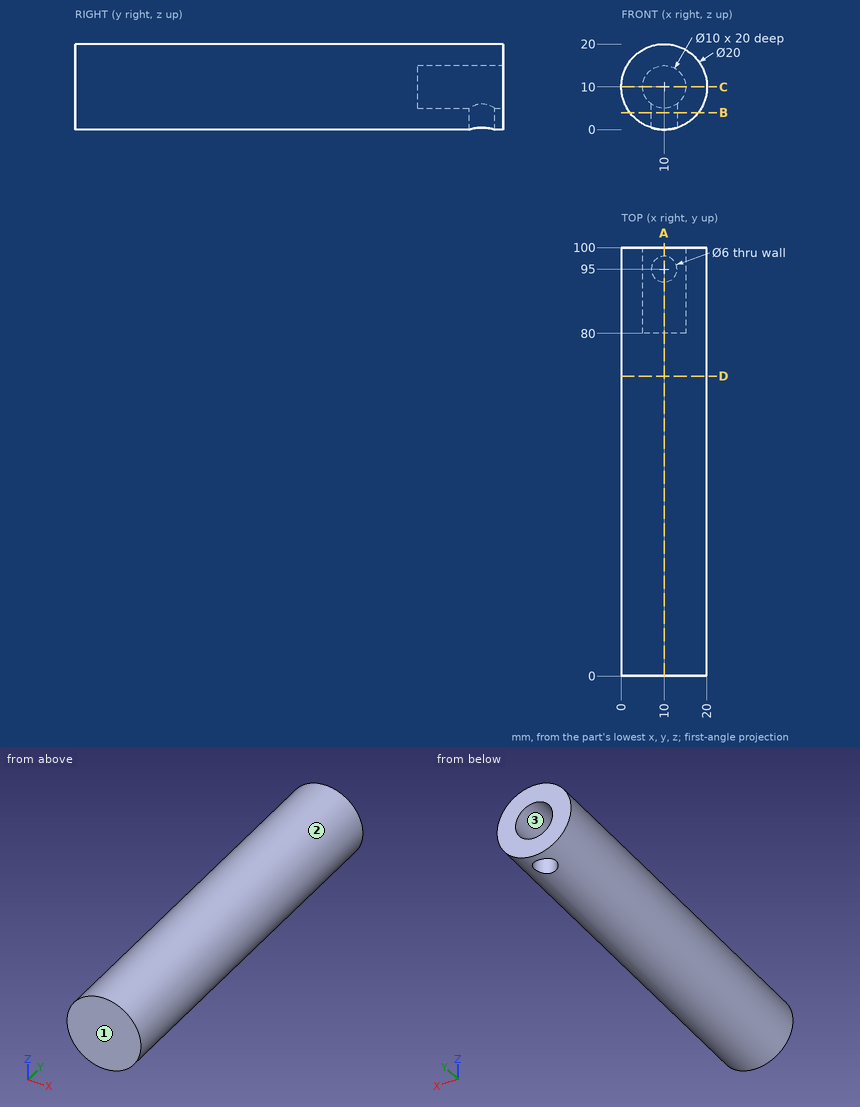
Design review of the part shown in the three views and the two pictorial views. Dimensions are in mm from the part's minimum x, y and z. Round coordinates to 2 decimals unless told otherwise and drop trailing zeros. Write each loop counter-clockwise with the first axis right and the second up, starting at its lowest first coordinate (ties: lowest second). Pieces come first, ordered by that corner, then holes.
Item 1: The part is to be moulded in two halves that separate along X. For the marked faces 1, 2 and 3, say which applies: +X half, -X half, draft (parallel to the pull), parting line (faces both ways), or undercut.
Item 2: We need section D-D on y = 70. Write out the cut boundary in (x, z), and give its area (3 significant figures).
Item 3: For probe 1 along Z at (x, y) = (10, 87.75); probe 2 along Z at (x, y) = (10, 92.5); probe 3 along Y at (x, z) = (9.5, 4.5), list the stretches that pass through material, from the lowest coordinate up.
Item 4: We need section B-B on z = 4. Write out the cut boundary in (x, y), and give its area (3 significant figures).
Item 5: Clearance check with flat-ended pins moving along their axes: pin 1 Ø8 at (x, y) = (2, 46.5) entering from +Z; pin 2 Ø2 at (x, y) = (8, 57) entering from +Z; pin 3 Ø6 at (y, z) = (42.5, 2.5) entering from +X. State where each tip first meets the part, or that it passes through.
Item 6: We need section A-A on x = 10. Write out the cut boundary in (y, z).
Item 7: We need section C-C on z = 10. Write out the cut boundary in (x, y), and give its area (3 significant figures).
Returned:
1. face 1: draft
1. face 2: parting line
1. face 3: undercut
2. outline: circle Ø20 at (10, 10)
2. area: 314 mm2
3. probe 1: z = 0 to 5, 15 to 20
3. probe 2: z = 15 to 20
3. probe 3: y = 0 to 92.04, 97.96 to 100
4. outline: (2, 0) - (18, 0) - (18, 100) - (2, 100) - close; hole circle Ø6 at (10, 95)
4. area: 1,570 mm2
5. pin 1: stops at z = 19.17
5. pin 2: stops at z = 19.95
5. pin 3: stops at x = 18.93
6. outline: (0, 0) - (92, 0) - (92, 5) - (80, 5) - (80, 15) - (100, 15) - (100, 20) - (0, 20) - close; (98, 0) - (100, 0) - (100, 5) - (98, 5) - close
7. outline: (0, 0) - (20, 0) - (20, 100) - (15, 100) - (15, 80) - (5, 80) - (5, 100) - (0, 100) - close
7. area: 1,800 mm2
